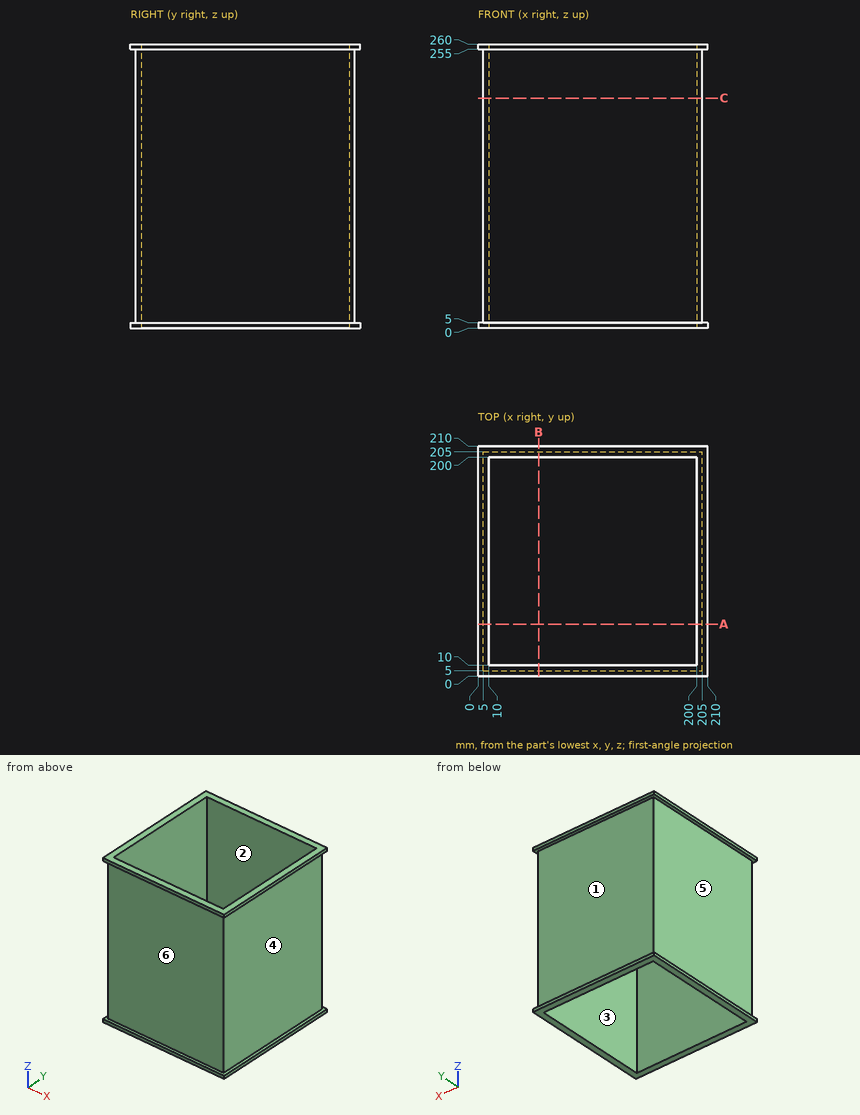
Design review of the part shown in the three views and the two pictorial views. Dimensions are in mm from the part's minimum x, y and z. A direction names the side the tool comes from. Round coordinates to 2 decimals unless told otherwise and drop trailing zeros. Order: outer loops, then holes, each group sorted by start corner. A loop starts at its lowest first (then second) coordinate and runs counter-clockwise, first axis right, second up.
Item 1: Add section C-C, the plane z = 210.5. State the section outline as (x, y) points, and give its area (3 significant figures).
Working result:
outline: (5, 5) - (205, 5) - (205, 205) - (5, 205) - close; hole (10, 10) - (200, 10) - (200, 200) - (10, 200) - close
area: 3,900 mm2
Item 2: For pin 1 (8 mm diameter, centred on x = 79, z = 74, fed in from -Y); pin 2 (5 mm diameter, centred on x = 114.5, z = 166.5, fed in from +Y); pin 3 (3 mm diameter, centred on y = 93, z = 126, fed in from +X), all flat-tipped, find the tip position at first contact; note any pin that passes through.
Working result:
pin 1: stops at y = 5
pin 2: stops at y = 205
pin 3: stops at x = 205
Item 3: To check wall thickness, follow probe 1 along Y at (x, z) = (163, 15.5). State the ranges of the line that lie inside material, in increasing order.
Working result:
probe 1: y = 5 to 10, 200 to 205
Item 4: Draft analysis for pull direction Z (two halves, no side actions). For the marked faces 1 and 2, state which applies: released by +Z, released by -Z, zero draft, split by the parting line, or undercut.
Working result:
face 1: undercut
face 2: zero draft
Item 5: Add section A-A, the plane y = 47.5. State the section outline as (x, z) points, and give its area (3 significant figures).
Working result:
outline: (0, 0) - (10, 0) - (10, 260) - (0, 260) - (0, 255) - (5, 255) - (5, 5) - (0, 5) - close; (200, 0) - (210, 0) - (210, 5) - (205, 5) - (205, 255) - (210, 255) - (210, 260) - (200, 260) - close
area: 2,700 mm2
Item 6: Machinability: for the marked faces 3, 4, 5 and 6, which of the approach directions +Z, -Z, +X, -X, +Y, -Y give a long, thin tool a straight path to every point of the face, cutting with its end or side? Answer none if there is none.
Working result:
face 3: +Z, -Z
face 4: +X, +Y, -Y
face 5: -X, +Y, -Y
face 6: +X, -X, -Y
